from build123d import *

# Parameters (mm, degrees)
EXTRUDE_1_DEPTH     = 3
SKETCH_2_R          = 1.5
CUT_EXTRUDE_1_DEPTH = 3
SKETCH_3_R          = 15
SKETCH_3_R_2        = 1.5
CUT_EXTRUDE_2_DEPTH = 10
SKETCH_4_W          = 90
SKETCH_4_H          = 80
CUT_EXTRUDE_3_DEPTH = 3
FILLET_3_R          = 6
CHAMFER_1_SIZE      = 8
SKETCH_7_R          = 1.5
CUT_EXTRUDE_6_DEPTH = 10
CHAMFER_2_SIZE      = 25
SKETCH_8_R          = 1.5
CUT_EXTRUDE_7_DEPTH = 10
SKETCH_9_R          = 1.5
CUT_EXTRUDE_8_DEPTH = 10


with BuildPart() as part:
    # 草图1 → 凸台-拉伸1 (new body)
    with BuildSketch(Plane(origin=(0, 0, 0), x_dir=(1, 0, 0), z_dir=(0, 1, 0))):
        Polygon((-50, -51), (-50, -105), (50, -105), (50, -51), (145, -51), (145, 51), (50, 51), (50, 105), (-50, 105), (-50, 51), (-145, 51), (-145, -51), align=None)
    extrude(amount=EXTRUDE_1_DEPTH)

    # 草图2 → 切除-拉伸1 (cut)
    with BuildSketch(Plane(origin=(0, 3, 0), x_dir=(1, 0, 0), z_dir=(0, 1, 0))):
        with Locations(Location((111, 42, 0), (0, 0, 270))):
            Circle(SKETCH_2_R)
        with Locations(Location((81, 42, 0), (0, 0, 270))):
            Circle(SKETCH_2_R)
        with Locations(Location((81, 18, 0), (0, 0, 270))):
            Circle(SKETCH_2_R)
        with Locations(Location((111, 18, 0), (0, 0, 270))):
            Circle(SKETCH_2_R)
        with Locations(Location((111, -18, 0), (0, 0, 90))):
            Circle(SKETCH_2_R)
        with Locations(Location((111, -42, 0), (0, 0, 90))):
            Circle(SKETCH_2_R)
        with Locations(Location((81, -18, 0), (0, 0, 90))):
            Circle(SKETCH_2_R)
        with Locations(Location((81, -42, 0), (0, 0, 90))):
            Circle(SKETCH_2_R)
        with Locations(Location((-81, -42, 0), (0, 0, 270))):
            Circle(SKETCH_2_R)
        with Locations(Location((-81, -18, 0), (0, 0, 270))):
            Circle(SKETCH_2_R)
        with Locations(Location((-111, -42, 0), (0, 0, 270))):
            Circle(SKETCH_2_R)
        with Locations(Location((-111, -18, 0), (0, 0, 270))):
            Circle(SKETCH_2_R)
        with Locations(Location((-111, 18, 0), (0, 0, 90))):
            Circle(SKETCH_2_R)
        with Locations(Location((-81, 18, 0), (0, 0, 90))):
            Circle(SKETCH_2_R)
        with Locations(Location((-81, 42, 0), (0, 0, 90))):
            Circle(SKETCH_2_R)
        with Locations(Location((-111, 42, 0), (0, 0, 90))):
            Circle(SKETCH_2_R)
    extrude(amount=-CUT_EXTRUDE_1_DEPTH, mode=Mode.SUBTRACT)

    # 草图3 → 切除-拉伸2 (cut)
    with BuildSketch(Plane(origin=(0, 3, 0), x_dir=(1, 0, 0), z_dir=(0, 1, 0))):
        with Locations(Location((0, 77, 0), (0, 0, 270))):
            Circle(SKETCH_3_R)
        with Locations(Location((0, -78, 0), (0, 0, 270))):
            Circle(SKETCH_3_R)
        with Locations(Location((15.11, -58, 0), (0, 0, 270))):
            Circle(SKETCH_3_R_2)
        with Locations(Location((15.11, -98, 0), (0, 0, 270))):
            Circle(SKETCH_3_R_2)
        with Locations(Location((-34.89, -98, 0), (0, 0, 270))):
            Circle(SKETCH_3_R_2)
        with Locations(Location((-34.89, -58, 0), (0, 0, 270))):
            Circle(SKETCH_3_R_2)
        with Locations(Location((15.11, 97, 0), (0, 0, 270))):
            Circle(SKETCH_3_R_2)
        with Locations(Location((15.11, 57, 0), (0, 0, 270))):
            Circle(SKETCH_3_R_2)
        with Locations(Location((-34.89, 57, 0), (0, 0, 270))):
            Circle(SKETCH_3_R_2)
        with Locations(Location((-34.89, 97, 0), (0, 0, 270))):
            Circle(SKETCH_3_R_2)
    extrude(amount=-CUT_EXTRUDE_2_DEPTH, mode=Mode.SUBTRACT)

    # 草图4 → 切除-拉伸3 (cut)
    with BuildSketch(Plane(origin=(0, 3, 0), x_dir=(1, 0, 0), z_dir=(0, 1, 0))):
        Rectangle(SKETCH_4_W, SKETCH_4_H)
    extrude(amount=-CUT_EXTRUDE_3_DEPTH, mode=Mode.SUBTRACT)

    # 圆角3
    fillet_3_edges = [part.edges().sort_by_distance(p)[0] for p in [
        (-145, 1.5, 51),
        (-145, 1.5, -51),
        (-50, 1.5, -105),
        (50, 1.5, -105),
        (145, 1.5, -51),
        (145, 1.5, 51),
        (50, 1.5, 105),
        (-50, 1.5, 105),
    ]]
    fillet(fillet_3_edges, radius=FILLET_3_R)

    # 倒角1
    chamfer_1_edges = [part.edges().sort_by_distance(p)[0] for p in [
        (-50, 1.5, 51),
        (-50, 1.5, -51),
        (50, 1.5, -51),
        (50, 1.5, 51),
    ]]
    chamfer(chamfer_1_edges, length=CHAMFER_1_SIZE)

    # 草图7 → 切除-拉伸6 (cut)
    with BuildSketch(Plane(origin=(0, 3, 0), x_dir=(1, 0, 0), z_dir=(0, 1, 0))):
        with Locations(Location((141.5, 29, 0), (0, 0, 270))):
            Circle(SKETCH_7_R)
        with Locations(Location((133.5, 29, 0), (0, 0, 270))):
            Circle(SKETCH_7_R)
        with Locations(Location((132, 15, 0), (0, 0, 270))):
            Circle(SKETCH_7_R)
        with Locations(Location((132, -45, 0), (0, 0, 270))):
            Circle(SKETCH_7_R)
        with Locations(Location((51, 32.5, 0), (0, 0, 270))):
            Circle(SKETCH_7_R)
        with Locations(Location((51, -32.5, 0), (0, 0, 270))):
            Circle(SKETCH_7_R)
        with Locations(Location((71, 32.5, 0), (0, 0, 270))):
            Circle(SKETCH_7_R)
        with Locations(Location((71, -32.5, 0), (0, 0, 270))):
            Circle(SKETCH_7_R)
        with BuildLine():
            Line((-65, -20), (-65, 20))
            ThreePointArc((-65, 20), (-60, 25), (-55, 20))
            Line((-55, 20), (-55, -20))
            ThreePointArc((-55, -20), (-60, -25), (-65, -20))
        make_face()
        with BuildLine():
            Line((65, -20), (65, 20))
            ThreePointArc((65, 20), (60, 25), (55, 20))
            Line((55, 20), (55, -20))
            ThreePointArc((55, -20), (60, -25), (65, -20))
        make_face()
        with BuildLine():
            Line((-141, -15), (-141, 15))
            ThreePointArc((-141, 15), (-137, 19), (-133, 15))
            Line((-133, 15), (-133, -15))
            ThreePointArc((-133, -15), (-137, -19), (-141, -15))
        make_face()
        with BuildLine():
            Line((128, -28), (128, 2))
            ThreePointArc((128, 2), (132, 6), (136, 2))
            Line((136, 2), (136, -28))
            ThreePointArc((136, -28), (132, -32), (128, -28))
        make_face()
    extrude(amount=-CUT_EXTRUDE_6_DEPTH, mode=Mode.SUBTRACT)

    # 倒角2
    chamfer_2_edges = [part.edges().sort_by_distance(p)[0] for p in [
        (45, 1.5, -40),
        (45, 1.5, 40),
        (-45, 1.5, 40),
        (-45, 1.5, -40),
    ]]
    chamfer(chamfer_2_edges, length=CHAMFER_2_SIZE)

    # 草图8 → 切除-拉伸7 (cut)
    with BuildSketch(Plane(origin=(0, 3, 0), x_dir=(1, 0, 0), z_dir=(0, 1, 0))):
        with Locations(Location((-127.5, 47, 0), (0, 0, 270))):
            Circle(SKETCH_8_R)
        with Locations(Location((-127.5, -11, 0), (0, 0, 270))):
            Circle(SKETCH_8_R)
    extrude(amount=-CUT_EXTRUDE_7_DEPTH, mode=Mode.SUBTRACT)

    # 草图9 → 切除-拉伸8 (cut)
    with BuildSketch(Plane(origin=(0, 3, 0), x_dir=(1, 0, 0), z_dir=(0, 1, 0))):
        with Locations(Location((43.343145751, 44, 0), (0, 0, 270))):
            Circle(SKETCH_9_R)
        with Locations(Location((49, 38.343145751, 0), (0, 0, 270))):
            Circle(SKETCH_9_R)
        with Locations(Location((49, -38.343145751, 0), (0, 0, 270))):
            Circle(SKETCH_9_R)
        with Locations(Location((43.343145751, -44, 0), (0, 0, 270))):
            Circle(SKETCH_9_R)
        with Locations(Location((-43.343145751, -44, 0), (0, 0, 270))):
            Circle(SKETCH_9_R)
        with Locations(Location((-49, -38.343145751, 0), (0, 0, 270))):
            Circle(SKETCH_9_R)
        with Locations(Location((-49, 38.343145751, 0), (0, 0, 270))):
            Circle(SKETCH_9_R)
        with Locations(Location((-43.343145751, 44, 0), (0, 0, 270))):
            Circle(SKETCH_9_R)
    extrude(amount=-CUT_EXTRUDE_8_DEPTH, mode=Mode.SUBTRACT)


solid = part.part
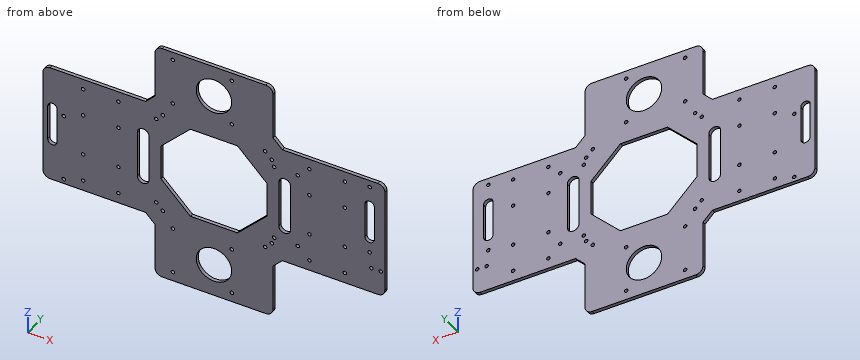
The listing builds one solid part. Answer for the finished solid, in the listing's coordinates (mm). Round coordinates to 2 decimals unless told otherwise and drop trailing zeros. Order: outer loops, then holes, each group sorted by start corner. A loop starts at its lowest first (then second) coordinate and runs counter-clockwise, first axis right, second up. Notation, with made-up numbers: (-31.75, -25.5) - (-15.75, -25.5) arc R8 ccw to (-15.75, -14.5) - close; hole circle Ø4 at (76, 10.5). An arc over 180 degrees is marked (long way). Write item = value, one per line. Start each with the question number.
1) Section B-B, the plane x = 95 is taken. Write down the section's boundary in (y, z).
2) Section A-A, the plane z = -73.5 is taken. Write down the section's boundary in (x, y), plus the area to 3 significant figures.
3) Straight lines are drawn through the part: L1, parallel to Z at x = 111, y = 1.95; L2, parallel to X at y = 2, z = -42; L3, parallel to Z at x = -127.5, y = 1. For each, find the intervals that lie inside material, in ascending order.
4) Section C-C, the plane y = 1.15 is taken. Count the separate pieces of the cut face and the enclosed holes in it, plus the area to 3 significant figures.
Results list:
q1.outline = (0, -51) - (3, -51) - (3, 51) - (0, 51) - close
q2.outline = (-50, 0) - (-14.59, 0) - (-14.59, 3) - (-50, 3) - close; (14.59, 0) - (50, 0) - (50, 3) - (14.59, 3) - close
q2.area = 212 mm^2
q3.L1 = -51 to -43.5, -40.5 to -19.5, -16.5 to 16.5, 19.5 to 40.5, 43.5 to 51
q3.L2 = -145 to -112.5, -109.5 to -82.5, -79.5 to 79.5, 82.5 to 109.5, 112.5 to 145
q3.L3 = -51 to -48.5, -45.5 to 9.5, 12.5 to 51
q4.separate_pieces = 1
q4.enclosed_holes = 49
q4.area = 31,200 mm^2
